Could you check a few things on this drawing? It's one solid part, dimensions in mm from its lowest x, y, z. A direction names the side the tool comes from. Coordinates: 2 decimals unless noted, no trailing zeros. Order: outer loops, then holes, each group sorted by start corner. A loop starts at its lowest first (then second) coordinate and runs counter-clockwise, first axis right, second up. Notation, with made-up numbers: M 12,64.5 L 24,64.5 A11 ccw 24,80.5 Z; hole C 82,79 d9. An arc over 180 degrees is marked long. One line per question, with ' | ' between items. Start each with the question number.
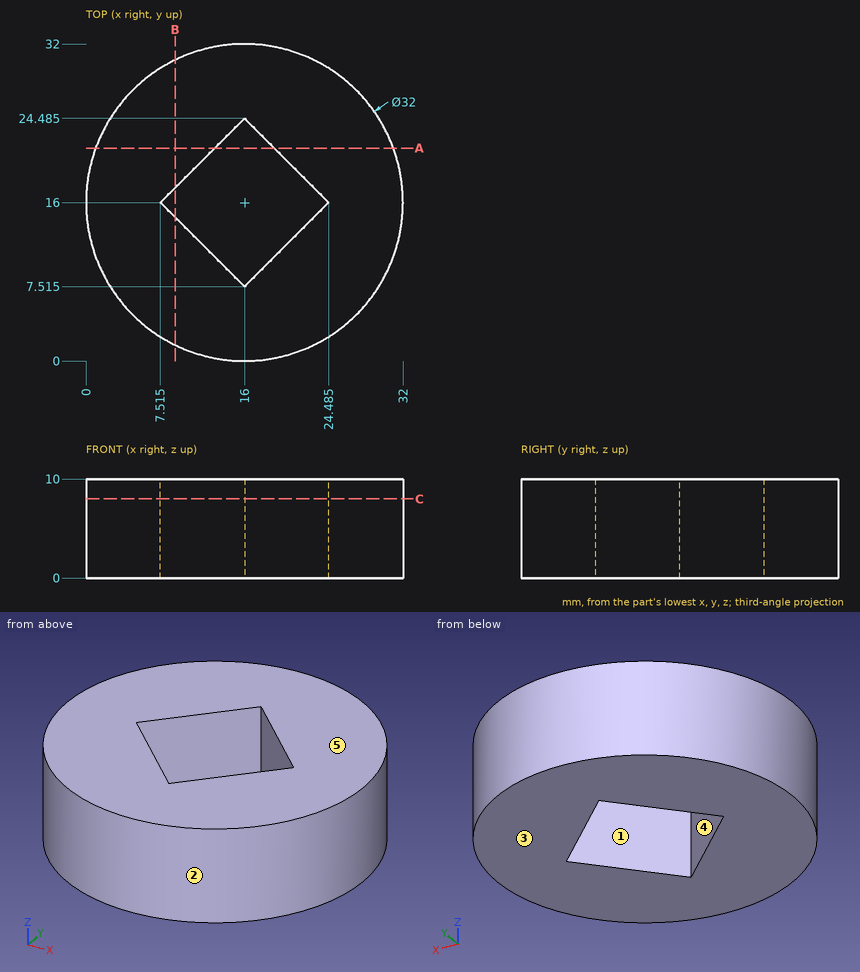
1. Imagine slicing it at A-A (y = 21.5). List the corners of the cut face in (x, z) for me (1 decimal), then the cut area to 3 significant figures.
2. Imagine slicing it at B-B (x = 9). List the corners of the cut face in (y, z) for me (1 decimal).
3. Imagine slicing it at C-C (z = 8). List the corners of the cut face in (x, y) for me (1 decimal).
4. Will these pins go through, and if not, where does the flat tip stop? pin 1 (1 mm diameter, centred on x = 23.5, y = 7, fed in from -Z); pin 2 (4 mm diameter, centred on x = 7.5, z = 8, fed in from -Y); pin 3 (1 mm diameter, centred on y = 5, z = 8, fed in from +X); pin 4 (6 mm diameter, centred on x = 4, z = 1.5, fed in from +Y).
5. Which directions (+Z, -Z, +X, -X, +Y, -Y) give clear straight access to the entire face, cutting with the end or side of a thin tool? Please do the marked faces 4 and 5.
6. We'd pull the mould along X, two halves only. Please class the marked faces 1, 2 and 3: released by +X, released by -X, zero draft, split by the parting line, or undercut.
7. I need wall thicknesses on line 1 (Y direction, x = 22.5, z = 3) (1 decimal); line 2 (X direction, y = 22, z = 2) (1 decimal). Which ranges of each line are inside material? Lowest first, please.
Entries:
1) outline: M 1,0 L 13,0 L 13,10 L 1,10 Z; M 19,0 L 31,0 L 31,10 L 19,10 Z | area: 241 mm²
2) outline: M 1.6,0 L 14.5,0 L 14.5,10 L 1.6,10 Z; M 17.5,0 L 30.4,0 L 30.4,10 L 17.5,10 Z
3) outline: C 16,16 d32; hole M 7.5,16 L 16,7.5 L 24.5,16 L 16,24.5 Z
4) pin 1: z = 0 | pin 2: y = 1.38 | pin 3: x = 28.07 | pin 4: y = 29.23
5) face 4: +Z, -Z | face 5: +Z, +X, -X, +Y, -Y
6) face 1: undercut | face 2: split by the parting line | face 3: zero draft
7) line 1: 1.4 to 14, 18 to 30.6 | line 2: 1.2 to 13.5, 18.5 to 30.8
